from build123d import *

# Parameters (mm, degrees)
SKETCH1_R             = 20
SKETCH1_R_2           = 10
SKETCH1_R_3           = 2
SKETCH1_R_4           = 2.5
BOSS_EXTRUDE1_DEPTH   = 5
BODY_MOVE_COPY1_ANGLE = 180


with BuildPart() as part:
    # Sketch1 → Boss-Extrude1 (new body)
    with BuildSketch(Plane(origin=(0, 0, 0), x_dir=(0, 0, -1), z_dir=(1, 0, 0))):
        Circle(SKETCH1_R)
        Circle(SKETCH1_R_2, mode=Mode.SUBTRACT)
        with Locations((-11, 11)):
            Circle(SKETCH1_R_3, mode=Mode.SUBTRACT)
        with Locations((11, 11)):
            Circle(SKETCH1_R_3, mode=Mode.SUBTRACT)
        with Locations((11, -11)):
            Circle(SKETCH1_R_3, mode=Mode.SUBTRACT)
        with Locations((-11, -11)):
            Circle(SKETCH1_R_3, mode=Mode.SUBTRACT)
        with Locations((-15, 0)):
            Circle(SKETCH1_R_4, mode=Mode.SUBTRACT)
    extrude(amount=BOSS_EXTRUDE1_DEPTH)


with BuildPart() as part_1:
    # Body-Move/Copy1: moved
    add(part.part.rotate(Axis((0, 0, 0), (0.7071067811865488, 0, 0.7071067811865462)), BODY_MOVE_COPY1_ANGLE))


solid = part_1.part
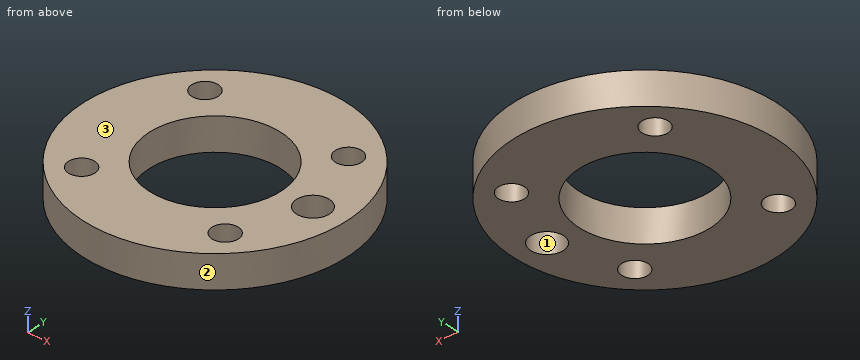
The listing builds one solid part. Answer for the finished solid, in the listing's coordinates (mm). Face numbers are marked on the shaded views. Round coordinates to 2 decimals unless told otherwise and drop trailing zeros. Order: outer loops, then holes, each group sorted by start corner. A loop starts at its lowest first (then second) coordinate and runs counter-clockwise, first axis right, second up. Notation, with made-up numbers: (62, -5.75) -> (97, -5.75) arc R26 ccw to (97, 31.25) -> close; hole circle Ø11 at (52.25, 6.25). An arc over 180 degrees is marked (long way). Put each result on its own line as item: value.
Q1. Section D-D, the plane x = 12 is taken. Write down the section's boundary in (y, z).
Results list:
outline: (-16, 0) -> (-12.73, 0) -> (-12.73, 5) -> (-16, 5) -> close; (-9.27, 0) -> (9.27, 0) -> (9.27, 5) -> (-9.27, 5) -> close; (12.73, 0) -> (16, 0) -> (16, 5) -> (12.73, 5) -> close
Q2. Each of these flat-tipped pins is pushed along its axis until it touches: P1, Ø4.5, axis at x = 15, y = 0, coming from the +Z side; P2, Ø1, axis at y = 7, z = 2, coming from the +X side. Where does it stop, or does it pass through?
Results list:
P1: through
P2: x = 18.91
Q3. Section C-C, the plane z = 1.95 is taken. Write down the section's boundary in (x, y).
Results list:
outline: circle Ø40 at (0, 0); hole circle Ø4 at (-11, -11); hole circle Ø4 at (-11, 11); hole circle Ø20 at (0, 0); hole circle Ø4 at (11, -11); hole circle Ø4 at (11, 11); hole circle Ø5 at (15, 0)
Q4. Section B-B, the plane x = 0 is taken. Write down the section's boundary in (y, z), and give its area (3 significant figures).
Results list:
outline: (-20, 0) -> (-10, 0) -> (-10, 5) -> (-20, 5) -> close; (10, 0) -> (20, 0) -> (20, 5) -> (10, 5) -> close
area: 100 mm^2
Q5. Consider line 1 along Y through (x, z) = (-11, 3.25); line 2 along X through (y, z) = (2, 4.75); line 3 along Y through (x, z) = (-5, 3.5). Determine where each line is inside the solid, lowest interval first.
Results list:
line 1: -16.7 to -13, -9 to 9, 13 to 16.7
line 2: -19.9 to -9.8, 9.8 to 13.5, 16.5 to 19.9
line 3: -19.36 to -8.66, 8.66 to 19.36
Q6. Section A-A, the plane y = 0 is taken. Write down the section's boundary in (x, z), and give its area (3 significant figures).
Results list:
outline: (-20, 0) -> (-10, 0) -> (-10, 5) -> (-20, 5) -> close; (10, 0) -> (12.5, 0) -> (12.5, 5) -> (10, 5) -> close; (17.5, 0) -> (20, 0) -> (20, 5) -> (17.5, 5) -> close
area: 75.0 mm^2
Q7. Determine the mould class of the marked faces 1, 2 and 3 for opening direction Y: pulls with the +Y half, pulls with the -Y half, needs draft (parallel to the pull), parting line crosses it, or undercut.
Results list:
face 1: undercut
face 2: parting line crosses it
face 3: needs draft
